Geometry: final body of the model. Coordinates: model frame, mm. A direction names the side the tool comes from. Give positions to 0.01 mm unless a question says otherwise; leave off trailing zeros. Write each loop counter-clockwise with the first axis right and the second up, starting at its lowest first coordinate (ties: lowest second). Pieces come first, ordered by that corner, then holes. Notation, with made-up numbers: M -25.5,16 L 4.5,16 A29 cw 4.5,46 Z; hole C 75.25,70.25 d6. An arc over 180 degrees is marked long. Use one line per item in the form item = value. Start each with the question number.
Item 1: Section query B-B on x = -3. Return loops of the section in (y, z).
Item 2: Section query A-A on y = -35. Return loops of the section in (x, z), then the cut area to 3 significant figures.
Item 3: Access query for faces 4 (the flat face through (-1, 12, 0)), 5 (the cylindrical face through (5.433, 9.565, 1.479)). Directions: +Z, -Z, +X, -X, +Y, -Y. A direction counts if a zero-diameter tool reaches every point of the face in a straight line with its end or side. Return the directions, or none.
Item 4: Pull-direction query (Y, two-part tool) for faces 1 (the cylindrical face through (-0.37, -50.32, 1.48)), 2 (the cylindrical face through (-2.81, -47.64, 1.48)), 3 (the cylindrical face through (0.37, 50.32, 1.48)); classes: released by +Y, released by -Y, zero draft, split by the parting line, or undercut.
Item 5: Section query C-C on y = -17.5. Return loops of the section in (x, z).
Item 6: Material intervals for line 1 along Y through (x, z) = (0.5, 1.3); line 2 along X through (y, z) = (15, 0.9); line 3 along X through (y, z) = (-25.5, 0.85), sorted ascending. Write a range as from..to.
Item 7: Section query D-D on x = 25.5. Return loops of the section in (y, z).
Item 8: Contact query for flat-ended pins moving along their axis: P1, Ø1, axis at y = -32.5, z = 1, coming from the -X side; P2, Ø20.5, axis at x = 0, y = -35, coming from the -Z side. Output: stop coordinate, or through.
from build123d import *

# Parameters (mm, degrees)
F0_R     = 12.95
F1_DEPTH = 3


with BuildPart() as f1:
    # F0 (on Top) → F1 (new body)
    with BuildSketch(Plane.XY):
        with BuildLine():
            ThreePointArc((42.56921, 0), (43.582425, 25.162325), (21.284605, 36.866017))
            ThreePointArc((21.284605, 36.866017), (0, 50.32465), (-21.284605, 36.866017))
            ThreePointArc((-21.284605, 36.866017), (-43.582425, 25.162325), (-42.56921, 0))
            ThreePointArc((-42.56921, 0), (-43.582425, -25.162325), (-21.284605, -36.866017))
            ThreePointArc((-21.284605, -36.866017), (0, -50.32465), (21.284605, -36.866017))
            ThreePointArc((21.284605, -36.866017), (43.582425, -25.162325), (42.56921, 0))
        make_face()
        with Locations((0, -35)):
            Circle(F0_R, mode=Mode.SUBTRACT)
        with Locations((-30.310889, -17.5)):
            Circle(F0_R, mode=Mode.SUBTRACT)
        with Locations((30.310889, -17.5)):
            Circle(F0_R, mode=Mode.SUBTRACT)
        with Locations((-30.310889, 17.5)):
            Circle(F0_R, mode=Mode.SUBTRACT)
        with BuildLine():
            ThreePointArc((9.393643, 5.72359), (9.526279, 5.5), (9.653595, 5.273338))
            ThreePointArc((9.653595, 5.273338), (11, 0), (9.653595, -5.273338))
            ThreePointArc((9.653595, -5.273338), (9.526279, -5.5), (9.393643, -5.72359))
            ThreePointArc((9.393643, -5.72359), (5.5, -9.526279), (0.259953, -10.996928))
            ThreePointArc((0.259953, -10.996928), (0, -11), (-0.259953, -10.996928))
            ThreePointArc((-0.259953, -10.996928), (-5.5, -9.526279), (-9.393643, -5.72359))
            ThreePointArc((-9.393643, -5.72359), (-9.526279, -5.5), (-9.653595, -5.273338))
            ThreePointArc((-9.653595, -5.273338), (-11, 0), (-9.653595, 5.273338))
            ThreePointArc((-9.653595, 5.273338), (-9.526279, 5.5), (-9.393643, 5.72359))
            ThreePointArc((-9.393643, 5.72359), (-5.5, 9.526279), (-0.259953, 10.996928))
            ThreePointArc((-0.259953, 10.996928), (0, 11), (0.259953, 10.996928))
            ThreePointArc((0.259953, 10.996928), (5.5, 9.526279), (9.393643, 5.72359))
        make_face(mode=Mode.SUBTRACT)
        with Locations((0, 35)):
            Circle(F0_R, mode=Mode.SUBTRACT)
        with Locations((30.310889, 17.5)):
            Circle(F0_R, mode=Mode.SUBTRACT)
    extrude(amount=F1_DEPTH)


solid = f1.part
Answer sheet:
q1.outline = M -50.13,0 L -47.6,0 L -47.6,3 L -50.13,3 Z; M -22.4,0 L -10.58,0 L -10.58,3 L -22.4,3 Z; M 10.58,0 L 22.4,0 L 22.4,3 L 10.58,3 Z; M 47.6,0 L 50.13,0 L 50.13,3 L 47.6,3 Z
q2.outline = M -32.55,0 L -12.95,0 L -12.95,3 L -32.55,3 Z; M 12.95,0 L 32.55,0 L 32.55,3 L 12.95,3 Z
q2.area = 118 mm2
q3.face_4 = -Z, +X, -X, +Y, -Y
q3.face_5 = +Z, -Z
q4.face_1 = released by -Y
q4.face_2 = undercut
q4.face_3 = released by +Y
q5.outline = M -46.38,0 L -43.26,0 L -43.26,3 L -46.38,3 Z; M -17.36,0 L 17.36,0 L 17.36,3 L -17.36,3 Z; M 43.26,0 L 46.38,0 L 46.38,3 L 43.26,3 Z
q6.line_1 = -50.32..-47.94, -22.06..-10.99, 10.99..22.06, 47.94..50.32
q6.line_2 = -46.68..-43.02, -17.6..17.6, 43.02..46.68
q6.line_3 = -43.38..-40.49, -20.13..-8.8, 8.8..20.13, 40.49..43.38
q7.outline = M -36.83,0 L -29.52,0 L -29.52,3 L -36.83,3 Z; M -5.48,0 L 5.48,0 L 5.48,3 L -5.48,3 Z; M 29.52,0 L 36.83,0 L 36.83,3 L 29.52,3 Z
q8.P1 = -37.62
q8.P2 = through
